from build123d import *

# Parameters (mm, degrees)
EXTRUDE_1_DEPTH     = 3
SKETCH_2_R          = 1.45
SKETCH_2_R_2        = 11
CUT_EXTRUDE_1_DEPTH = 5


with BuildPart() as part:
    # 草图1 → 凸台-拉伸1 (new body)
    with BuildSketch(Plane.XY):
        with BuildLine():
            Line((-12.500001384, 20), (12.499999997, 20))
            ThreePointArc((12.499999997, 20), (17.803300858, 17.80330086), (20, 12.5))
            Line((20, 12.5), (20, -12.5))
            ThreePointArc((20, -12.5), (17.803300859, -17.803300859), (12.5, -20))
            Line((12.5, -20), (-12.5, -20))
            ThreePointArc((-12.5, -20), (-17.80330064, -17.803301077), (-20, -12.500000618))
            Line((-20, -12.500000618), (-20, 12.5))
            ThreePointArc((-20, 12.5), (-17.803301348, 17.80330037), (-12.500001384, 20))
        make_face()
    extrude(amount=EXTRUDE_1_DEPTH)

    # 草图2 → 切除-拉伸1 (cut)
    with BuildSketch(Plane.XY):
        with Locations((15.5, 15.5)):
            Circle(SKETCH_2_R)
        with Locations(Location((-15.5, 15.5, 0), (0, 0, 180))):
            Circle(SKETCH_2_R)
        with Locations(Location((15.5, -15.5, 0), (0, 0, 180))):
            Circle(SKETCH_2_R)
        with Locations((-15.5, -15.5)):
            Circle(SKETCH_2_R)
        with Locations((0, 15)):
            Circle(SKETCH_2_R)
        with Locations((14, 0)):
            Circle(SKETCH_2_R)
        with Locations((-7, -12.124355653)):
            Circle(SKETCH_2_R)
        with Locations((-12.990381057, -7.5)):
            Circle(SKETCH_2_R)
        with Locations((12.990381057, -7.5)):
            Circle(SKETCH_2_R)
        with Locations((-7, 12.124355653)):
            Circle(SKETCH_2_R)
        Circle(SKETCH_2_R_2)
    extrude(amount=CUT_EXTRUDE_1_DEPTH, mode=Mode.SUBTRACT)


solid = part.part
The model under review builds one solid part; all positions refer to its coordinate system, in mm. Coordinates: 2 decimals unless noted, no trailing zeros. Write each loop counter-clockwise with the first axis right and the second up, starting at its lowest first coordinate (ties: lowest second). Pieces come first, ordered by that corner, then holes. Notation, with made-up numbers: (56, 48) -> (61, 48) arc R35 cw to (61, 86) -> close; hole circle Ø3 at (54.25, -30). An arc over 180 degrees is marked (long way). Answer in a Markdown table with one row per item.
1. We need section A-A, the plane x = 0. State the section outline as (y, z) points.
Answers below:
| item | result |
|---|---|
| outline | (-20, 0) -> (-11, 0) -> (-11, 3) -> (-20, 3) -> close; (11, 0) -> (13.55, 0) -> (13.55, 3) -> (11, 3) -> close; (16.45, 0) -> (20, 0) -> (20, 3) -> (16.45, 3) -> close |
2. We need section D-D, the plane x = -7. State the section outline as (y, z) points.
Answers below:
| item | result |
|---|---|
| outline | (-20, 0) -> (-13.57, 0) -> (-13.57, 3) -> (-20, 3) -> close; (-10.67, 0) -> (-8.49, 0) -> (-8.49, 3) -> (-10.67, 3) -> close; (8.49, 0) -> (10.67, 0) -> (10.67, 3) -> (8.49, 3) -> close; (13.57, 0) -> (20, 0) -> (20, 3) -> (13.57, 3) -> close |
3. Draft analysis for pull direction X (two halves, no side actions). For faces 1 (the flat face through (-20, 0, 1)), 2 (the flat face through (20, 0, 1)), 3 (the cylindrical face through (14.33, -8.06, 1.48)), state which applies: +X half, -X half, draft (parallel to the pull), parting line (faces both ways), or undercut.
Answers below:
| item | result |
|---|---|
| face 1 | -X half |
| face 2 | +X half |
| face 3 | undercut |
4. We need section C-C, the plane y = 15. State the section outline as (x, z) points, and give its area (3 significant figures).
Answers below:
| item | result |
|---|---|
| outline | (-19.57, 0) -> (-16.86, 0) -> (-16.86, 3) -> (-19.57, 3) -> close; (-14.14, 0) -> (-1.45, 0) -> (-1.45, 3) -> (-14.14, 3) -> close; (1.45, 0) -> (14.14, 0) -> (14.14, 3) -> (1.45, 3) -> close; (16.86, 0) -> (19.57, 0) -> (19.57, 3) -> (16.86, 3) -> close |
| area | 92.4 mm^2 |
5. Wall thickness on probe 1 along X at (y, z) = (12, 1); probe 2 along Y at (x, z) = (-7, 2.15); probe 3 along X at (y, z) = (-15.5, 0.7): over which ranges is each line inside the solid? List them lowest first. Write a range as [from, to].
Answers below:
| item | result |
|---|---|
| probe 1 | x = [-20, -8.44], [-5.56, 20] |
| probe 2 | y = [-20, -13.57], [-10.67, -8.49], [8.49, 10.67], [13.57, 20] |
| probe 3 | x = [-19.37, -16.95], [-14.05, 14.05], [16.95, 19.37] |
6. We need section B-B, the plane x = 8.5. State the section outline as (y, z) points.
Answers below:
| item | result |
|---|---|
| outline | (-20, 0) -> (-6.98, 0) -> (-6.98, 3) -> (-20, 3) -> close; (6.98, 0) -> (20, 0) -> (20, 3) -> (6.98, 3) -> close |
